Part model, mm, in its own coordinate system. A direction names the side the tool comes from. Give positions to 0.01 mm unless a question says otherwise; leave off trailing zeros. Order: outer loops, then holes, each group sorted by start corner. A loop starts at its lowest first (then second) coordinate and runs counter-clockwise, first axis right, second up. Notation, with made-up numbers: M -29,27.5 L 18,27.5 A27 ccw 18,65.5 Z; hole C -28.75,23.5 d10. An arc over 180 degrees is marked long. One line per question, with ' | ' between items.
```python
from build123d import *

# Parameters (mm, degrees)
SKETCH_R      = 1.6
SKETCH_W      = 9
SKETCH_H      = 19
SKETCH_W_2    = 6.2
SKETCH_H_2    = 6.2
PAD_DEPTH     = 4
SKETCH001_R   = 3
SKETCH001_R_2 = 1.6
PAD001_DEPTH  = 1
SKETCH002_W   = 2
SKETCH002_H   = 4
POCKET_DEPTH  = 4.001


with BuildPart() as part:
    # Sketch → Pad (new body)
    with BuildSketch(Plane.XY):
        Polygon((-72, 51.5), (-37, 51.5), (-27.440693, 31), (27.440693, 31), (37, 51.5), (72, 51.5), (72, -51.5), (37, -51.5), (26.434474, -31.5), (-26.434474, -31.5), (-37, -51.5), (-72, -51.5), align=None)
        with Locations((65, 35)):
            Circle(SKETCH_R, mode=Mode.SUBTRACT)
        with Locations((65, -35)):
            Circle(SKETCH_R, mode=Mode.SUBTRACT)
        with Locations((-65, 35)):
            Circle(SKETCH_R, mode=Mode.SUBTRACT)
        with Locations((-65, -35)):
            Circle(SKETCH_R, mode=Mode.SUBTRACT)
        with Locations((-50, 35)):
            Rectangle(SKETCH_W, SKETCH_H, mode=Mode.SUBTRACT)
        with Locations((-50, -35)):
            Rectangle(SKETCH_W, SKETCH_H, mode=Mode.SUBTRACT)
        with Locations((50, 0)):
            Rectangle(SKETCH_W, SKETCH_H, mode=Mode.SUBTRACT)
        with Locations((-20, 20.9)):
            Rectangle(SKETCH_W_2, SKETCH_H_2, mode=Mode.SUBTRACT)
        with Locations((-20, 8.9)):
            Rectangle(SKETCH_W_2, SKETCH_H_2, mode=Mode.SUBTRACT)
        with Locations((-20, -20.9)):
            Rectangle(SKETCH_W_2, SKETCH_H_2, mode=Mode.SUBTRACT)
        with Locations((-20, -8.9)):
            Rectangle(SKETCH_W_2, SKETCH_H_2, mode=Mode.SUBTRACT)
    extrude(amount=PAD_DEPTH)

    # Sketch001 → Pad001 (new body)
    with BuildSketch(Plane.XY.offset(4)):
        with Locations((65, 35)):
            Circle(SKETCH001_R)
        with Locations((65, 35)):
            Circle(SKETCH001_R_2, mode=Mode.SUBTRACT)
        with Locations((-65, 35)):
            Circle(SKETCH001_R)
        with Locations((-65, 35)):
            Circle(SKETCH001_R_2, mode=Mode.SUBTRACT)
        with Locations((-65, -35)):
            Circle(SKETCH001_R)
        with Locations((-65, -35)):
            Circle(SKETCH001_R_2, mode=Mode.SUBTRACT)
        with Locations((65, -35)):
            Circle(SKETCH001_R)
        with Locations((65, -35)):
            Circle(SKETCH001_R_2, mode=Mode.SUBTRACT)
    extrude(amount=PAD001_DEPTH)

    # Sketch002 → Pocket (cut, through all)
    with BuildSketch(Plane.XY.offset(4)):
        with Locations((-42, 40.5)):
            Rectangle(SKETCH002_W, SKETCH002_H)
        with Locations((-42, 29.5)):
            Rectangle(SKETCH002_W, SKETCH002_H)
        with Locations((-58, 40.5)):
            Rectangle(SKETCH002_W, SKETCH002_H)
        with Locations((-58, 29.5)):
            Rectangle(SKETCH002_W, SKETCH002_H)
        with Locations((42, 5.5)):
            Rectangle(SKETCH002_W, SKETCH002_H)
        with Locations((58, 5.5)):
            Rectangle(SKETCH002_W, SKETCH002_H)
        with Locations((58, -5.5)):
            Rectangle(SKETCH002_W, SKETCH002_H)
        with Locations((42, -5.5)):
            Rectangle(SKETCH002_W, SKETCH002_H)
        with Locations((-42, -29.5)):
            Rectangle(SKETCH002_W, SKETCH002_H)
        with Locations((-58, -29.5)):
            Rectangle(SKETCH002_W, SKETCH002_H)
        with Locations((-42, -40.5)):
            Rectangle(SKETCH002_W, SKETCH002_H)
        with Locations((-58, -40.5)):
            Rectangle(SKETCH002_W, SKETCH002_H)
    extrude(amount=-POCKET_DEPTH, mode=Mode.SUBTRACT)


solid = part.part
```
1. Mould opens along X. For faces 4 (the flat face through (54, 51.5, 2)), 5 (the flat face through (43, 5, 2)) say: released by +X, released by -X, zero draft, split by the parting line, or undercut.
Worked out:
face 4: zero draft | face 5: undercut
2. Tool access for faces 1 (the flat face through (-54, -51.5, 2)), 2 (the flat face through (-45.5, -35, 2)), 3 (the flat face through (0, 31, 2)): list every direction of +Z, -Z, +X, -X, +Y, -Y with a clear straight run to the whole face (end or side of a thin tool).
Worked out:
face 1: +Z, -Z, +X, -X, -Y | face 2: +Z, -Z | face 3: +Z, -Z, +Y
3. Slice it at D-D on z = 2.1. Give the number of separate pieces and of enclosed holes in the cut face, then the cut area to 3 significant figures.
Worked out:
separate pieces: 1 | enclosed holes: 23 | area: 11,400 mm2
4. Slice it at B-B on x = -65. Give the cut face in (y, z), then the cut area to 3 significant figures.
Worked out:
outline: M -51.5,0 L -36.6,0 L -36.6,5 L -38,5 L -38,4 L -51.5,4 Z; M -33.4,0 L 33.4,0 L 33.4,5 L 32,5 L 32,4 L -32,4 L -32,5 L -33.4,5 Z; M 36.6,0 L 51.5,0 L 51.5,4 L 38,4 L 38,5 L 36.6,5 Z | area: 392 mm2
5. Slice it at A-A on y = -0.5. Give the cut face in (x, z).
Worked out:
outline: M -72,0 L 45.5,0 L 45.5,4 L -72,4 Z; M 54.5,0 L 72,0 L 72,4 L 54.5,4 Z
6. Drop flat-ended pins along their axis: pin 1 (1.5 mm diameter, centred on x = 34.5, y = 30, fed in from +Z); pin 2 (3 mm diameter, centred on x = -11.5, y = 34, fed in from -Z); pin 3 (8 mm diameter, centred on x = 14, y = -14.5, fed in from -Z). Give the stop position or say it passes through.
Worked out:
pin 1: stops at z = 4 | pin 2: passes through | pin 3: stops at z = 0
7. Probe L1, parallel to Y at x = 65, z = 3.4; L2, parallel to X at y = 28, z = 1.15; L3, parallel to X at y = -32.5, z = 3.4. List the from-to ranges inside material, lowest first. Write a range as from..to.
Worked out:
L1: y = -51.5..-36.6, -33.4..33.4, 36.6..51.5 | L2: x = -72..-59, -57..-54.5, -45.5..-43, -41..72 | L3: x = -72..-54.5, -45.5..-26.96, 26.96..72
8. Slice it at C-C on y = -35. Give the cut face in (x, z).
Worked out:
outline: M -72,0 L -66.6,0 L -66.6,5 L -68,5 L -68,4 L -72,4 Z; M -63.4,0 L -54.5,0 L -54.5,4 L -62,4 L -62,5 L -63.4,5 Z; M -45.5,0 L -28.28,0 L -28.28,4 L -45.5,4 Z; M 28.28,0 L 63.4,0 L 63.4,5 L 62,5 L 62,4 L 28.28,4 Z; M 66.6,0 L 72,0 L 72,4 L 68,4 L 68,5 L 66.6,5 Z
